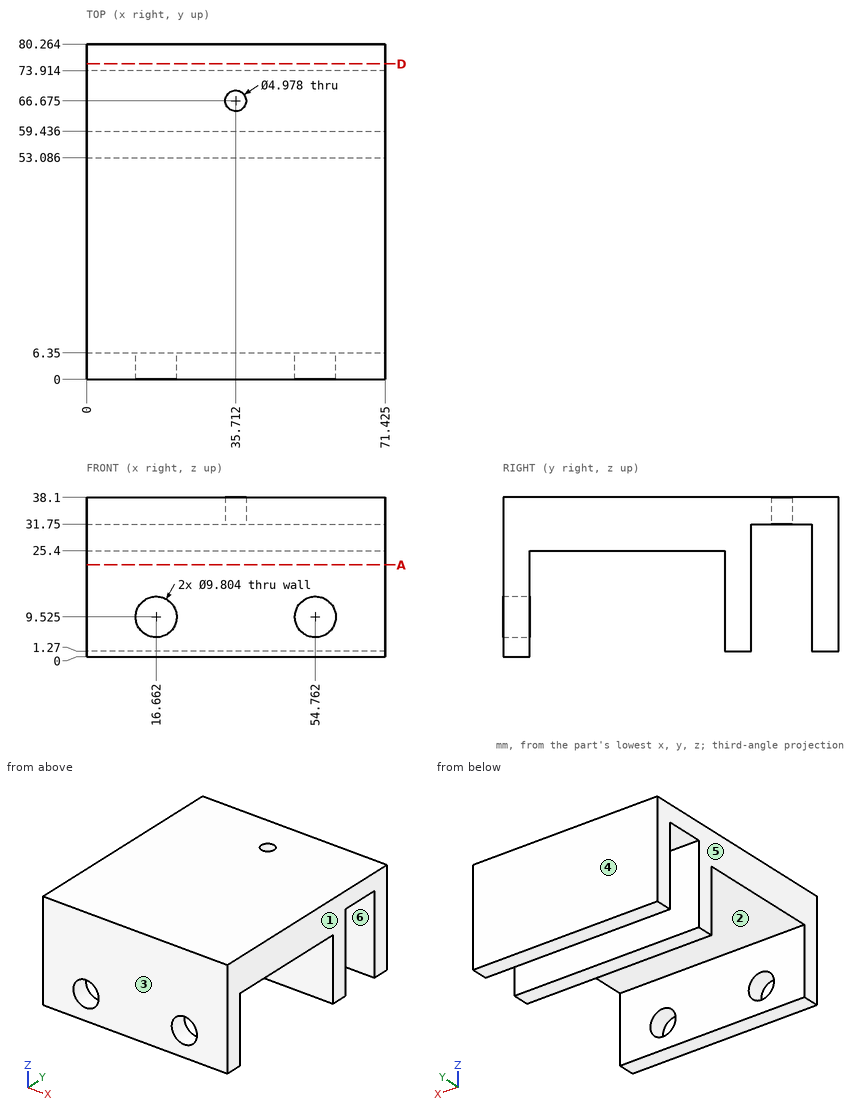
Check sheet for the drawn part. Datum: minimum x, y, z corner. Units: mm. A direction names the side the tool comes from. Round coordinates to 2 decimals unless told otherwise and drop trailing zeros. Order: outer loops, then holes, each group sorted by start corner. A loop starts at its lowest first (then second) coordinate and runs counter-clockwise, first axis right, second up.
(1) Access from +Z, -Z, +X, -X, +Y, -Y to the whole of each face (thin tool, end or side, straight path). Record for the marked faces 5 and 6.
(2) Go/stop test with flat-tipped pins: P1, Ø7, axis at x = 24, y = 69.5, coming from the -Z side; P2, Ø9, axis at x = 54.76, z = 9.52, coming from the -Y side; P3, Ø12, axis at x = 39, z = 8, coming from the -Y side; P4, Ø7, axis at x = 46.5, y = 58, coming from the -Z side. Record where each tip stops, or that it passes through.
(3) Cross-section at D-D, the plane y = 75.5. Enter the section's corners in (x, z) (1 decimal).
(4) Cross-section at A-A, the plane z = 22. State how many separate pieces and enclosed holes the cut face has, and give its area (3 significant figures).
(5) Draft check along Y on the marked faces 1, 2, 3 and 4. Enter one of: pulls with the +Y half, pulls with the -Y half, needs draft (parallel to the pull), parting line crosses it, or undercut.
(6) Scan lines: probe 1 along Y at (x, z) = (5.5, 15); probe 2 along Y at (x, z) = (38.5, 31). Record each from-to range of solid material in increasing order.
Check sheet entries:
1. face 5: +Z, -Z, -X, +Y, -Y
1. face 6: -Z, +X, -X
2. P1: stops at z = 31.75
2. P2: stops at y = 53.09
2. P3: stops at y = 0
2. P4: stops at z = 1.27
3. outline: (0, 1.3) - (71.4, 1.3) - (71.4, 38.1) - (0, 38.1) - close
4. separate pieces: 3
4. enclosed holes: 0
4. area: 1,360 mm2
5. face 1: needs draft
5. face 2: undercut
5. face 3: pulls with the -Y half
5. face 4: pulls with the +Y half
6. probe 1: y = 0 to 6.35, 53.09 to 59.44, 73.91 to 80.26
6. probe 2: y = 0 to 59.44, 73.91 to 80.26
